Autodesk Fusion 360 part; units mm, degrees
sketch "Sketch1" plane through (0, 0, 0) normal (0, 0, 1) x (1, 0, 0)
  line L0 (11, -40) -> (-11, -40)
  line L1 (-11, -42.5) -> (-11, 42.5)
  line L2 (-11, 40) -> (11, 40)
  line L3 (11, 42.5) -> (11, -42.5)
  line L4 (-13.5, -42.5) -> (-13.5, 42.5)
  line L5 (-13.5, 42.5) -> (13.5, 42.5)
  line L6 (13.5, 42.5) -> (13.5, -42.5)
  line L7 (13.5, -42.5) -> (-13.5, -42.5)
  dimension "d1" = 22
  dimension "d2" = 80
extrude "Extrude1" add sketch "Sketch1" along normal blind 3
extrude "Extrude2" add sketch "Sketch1" along normal blind 60 contours L3 L5 L6 L7 | L1 L4 L5 L7
fillet "Fillet1" radius 42.5 4 edges at (12.25, -42.5, 60) (-12.25, -42.5, 60) (12.25, 42.5, 60) (-12.25, 42.5, 60)
sketch "Sketch2" plane through (13.5, 0, 0) normal (1, 0, 0) x (0, 1, 0)
  arc A0 (42.5, 17.5) -> (-42.5, 17.5) centre (0, 17.5) ccw
  line L0 (-42.5, 17.5) -> (-42.5, 0)
  line L1 (-42.5, 0) -> (42.5, 0)
  line L2 (42.5, 0) -> (42.5, 17.5)
  circle A1 centre (0, 54) radius 5
  dimension "d10" = 10
extrude "Extrude3" add sketch "Sketch2" against normal blind 27 contours A1
Model file for the job. Use its own axes, mm. Round coordinates to 2 decimals unless told otherwise and drop trailing zeros. Write each loop counter-clockwise with the first axis right and the second up, starting at its lowest first coordinate (ties: lowest second). Pieces come first, ordered by that corner, then holes. Notation, with made-up numbers: (61.5, 14) - (110.5, 14) arc R15 ccw to (110.5, 26) - close; hole circle Ø5 at (-26, 86.25). An arc over 180 degrees is marked (long way). One line per item, written item: value.
(1) Cut at B-B, the plane x = 5.5. Give the cut face in (y, z), plus the area to 3 significant figures.
Values follow:
outline: (-42.5, 0) - (42.5, 0) - (42.5, 3) - (-42.5, 3) - close; circle Ø10 at (0, 54)
area: 334 mm²
(2) Cut at D-D, the plane z = 22. Give the cut face in (x, y).
Values follow:
outline: (-13.5, -42.26) - (-11, -42.26) - (-11, 42.26) - (-13.5, 42.26) - close; (11, -42.26) - (13.5, -42.26) - (13.5, 42.26) - (11, 42.26) - close
(3) Drop flat-ended pins along their axis: P1, Ø6, axis at x = 6, z = 39, coming from the -Y side; P2, Ø12, axis at x = 3, y = 22.5, coming from the +Z side. Give the stop position or say it passes through.
Values follow:
P1: passes through
P2: stops at z = 3
(4) Two-plate mould, pull along X, no slides. Class faces 1 (the flat face through (-13.5, -1, 23)), 2 (the cylindrical face through (0.154, -0.651, 58.957)), 3 (the cylindrical face through (12.232, -30.383, 47.222)): pulls with the +X half, pulls with the -X half, needs draft (parallel to the pull), parting line crosses it, or undercut.
Values follow:
face 1: pulls with the -X half
face 2: undercut
face 3: needs draft
(5) Cut at A-A, the plane z = 6. Give the cut face in (x, y), plus the area to 3 significant figures.
Values follow:
outline: (-13.5, -42.5) - (-11, -42.5) - (-11, 42.5) - (-13.5, 42.5) - close; (11, -42.5) - (13.5, -42.5) - (13.5, 42.5) - (11, 42.5) - close
area: 425 mm²
(6) Wall check: probe 1 along X at (y, z) = (30, 18); probe 2 along Z at (x, y) = (-7, 6); probe 3 along Z at (x, y) = (-2.5, -2). Give the ranges that are in metal, low to high.
Values follow:
probe 1: x = -13.5 to -11, 11 to 13.5
probe 2: z = 0 to 3
probe 3: z = 0 to 3, 49.42 to 58.58
(7) Cut at C-C, the plane y = -36. Give the cut face in (x, z), plus the area to 3 significant figures.
Values follow:
outline: (-13.5, 0) - (13.5, 0) - (13.5, 40.09) - (11, 40.09) - (11, 3) - (-11, 3) - (-11, 40.09) - (-13.5, 40.09) - close
area: 266 mm²
